CAD build for the part. Positions are in the model's coordinates, mm. A direction names the side the tool comes from. Round coordinates to 2 decimals unless told otherwise and drop trailing zeros. Order: outer loops, then holes, each group sorted by start corner. A loop starts at its lowest first (then second) coordinate and runs counter-clockwise, first axis right, second up. Notation, with made-up numbers: M -37,85 L 7,85 A24 cw 7,99 Z; hole C -35,-36 d11. An arc over 180 degrees is marked long. Answer as a JSON object with one key per item and string values.
```python
from build123d import *

# Parameters (mm, degrees)
SKETCH_R  = 1.5
SKETCH_W  = 2.1
SKETCH_H  = 24
PAD_DEPTH = 2
FILLET_R  = 1


with BuildPart() as part:
    # Sketch → Pad (new body)
    with BuildSketch(Plane.XY):
        Polygon((-11.7, 3.5), (-6.7, 3.5), (-6.7, -3.5), (6.7, -3.5), (6.7, 3.5), (11.7, 3.5), (11.7, -3.5), (11.7, -33.5), (-11.7, -33.5), (-11.7, -3.5), align=None)
        with Locations((-9.2, 0)):
            Circle(SKETCH_R, mode=Mode.SUBTRACT)
        with Locations((9.2, 0)):
            Circle(SKETCH_R, mode=Mode.SUBTRACT)
        with Locations((-5.45, -18.5)):
            Rectangle(SKETCH_W, SKETCH_H, mode=Mode.SUBTRACT)
        with Locations((5.45, -18.5)):
            Rectangle(SKETCH_W, SKETCH_H, mode=Mode.SUBTRACT)
    extrude(amount=PAD_DEPTH)

    # Fillet
    fillet_edges = [part.edges().sort_by_distance(p)[0] for p in [
        (-11.7, -33.5, 1),
        (11.7, -33.5, 1),
    ]]
    fillet(fillet_edges, radius=FILLET_R)


solid = part.part
```
Item 1: Saw through at C-C on z = 1.25. List the corners of the cut face in (x, y), and give its area (3 significant figures).
Worked answers:
{"outline": "M -11.7,-32.5 A1 ccw -10.7,-33.5 L 10.7,-33.5 A1 ccw 11.7,-32.5 L 11.7,3.5 L 6.7,3.5 L 6.7,-3.5 L -6.7,-3.5 L -6.7,3.5 L -11.7,3.5 Z; hole C -9.2,0 d3; hole M -6.5,-30.5 L -4.4,-30.5 L -4.4,-6.5 L -6.5,-6.5 Z; hole M 4.4,-30.5 L 6.5,-30.5 L 6.5,-6.5 L 4.4,-6.5 Z; hole C 9.2,0 d3", "area": "657 mm2"}
Item 2: Saw through at A-A on y = 0. List the corners of the cut face in (x, z), and give its area (3 significant figures).
Worked answers:
{"outline": "M -11.7,0 L -10.7,0 L -10.7,2 L -11.7,2 Z; M -7.7,0 L -6.7,0 L -6.7,2 L -7.7,2 Z; M 6.7,0 L 7.7,0 L 7.7,2 L 6.7,2 Z; M 10.7,0 L 11.7,0 L 11.7,2 L 10.7,2 Z", "area": "8.00 mm2"}
Item 3: Saw through at B-B on x = 9.2. List the corners of the cut face in (y, z), and give its area (3 significant figures).
Worked answers:
{"outline": "M -33.5,0 L -1.5,0 L -1.5,2 L -33.5,2 Z; M 1.5,0 L 3.5,0 L 3.5,2 L 1.5,2 Z", "area": "68.0 mm2"}
Item 4: 3-axis set-ups, long thin cutter, end or side, ignore diameter. For faces 1 (the flat face through (6.7, 0, 1)), 2 (the flat face through (-4.4, -19, 1)), 3 (the flat face through (0, -33.5, 1)): which of +Z, -Z, +X, -X, +Y, -Y reach the whole face in a straight line?
Worked answers:
{"face 1": "+Z, -Z, +Y", "face 2": "+Z, -Z", "face 3": "+Z, -Z, +X, -X, -Y"}
Item 5: Drop flat-ended pins along their axis: pin 1 Ø0.6 at (x, z) = (3, 0.5) entering from +Y; pin 2 Ø2.5 at (x, y) = (-9.2, 0) entering from -Z. Give the stop position or say it passes through.
Worked answers:
{"pin 1": "stops at y = -3.5", "pin 2": "passes through"}
Item 6: Wall check: line 1 along X through (y, z) = (-13, 0.5); line 2 along Y through (x, z) = (9.2, 0.85); line 3 along X through (y, z) = (-2, 1.25). Give the ranges that are in metal, low to high. Write a range as [from, to].
Worked answers:
{"line 1": "x = [-11.7, -6.5], [-4.4, 4.4], [6.5, 11.7]", "line 2": "y = [-33.5, -1.5], [1.5, 3.5]", "line 3": "x = [-11.7, -6.7], [6.7, 11.7]"}
Item 7: Two-plate mould, pull along X, no slides. Class faces 4 (the flat face through (9, 3.5, 1)), 5 (the flat face through (-6.7, 0, 1)), 6 (the cylindrical face through (11.399, -33.215, 1.014)): released by +X, released by -X, zero draft, split by the parting line, or undercut.
Worked answers:
{"face 4": "zero draft", "face 5": "undercut", "face 6": "released by +X"}
Item 8: Saw through at D-D on y = -17. List the corners of the cut face in (x, z).
Worked answers:
{"outline": "M -11.7,0 L -6.5,0 L -6.5,2 L -11.7,2 Z; M -4.4,0 L 4.4,0 L 4.4,2 L -4.4,2 Z; M 6.5,0 L 11.7,0 L 11.7,2 L 6.5,2 Z"}
